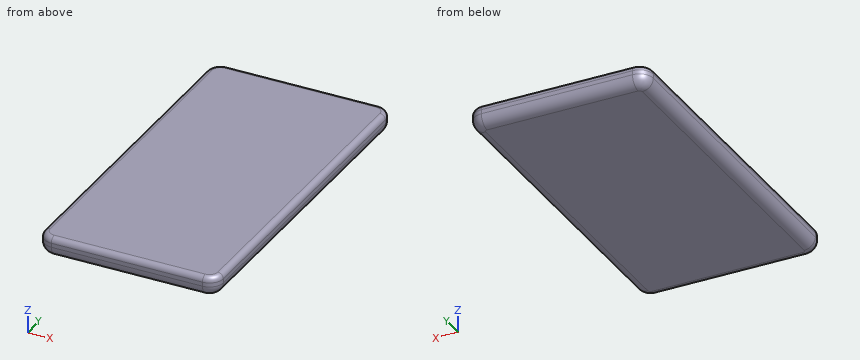
from build123d import *

# Parameters (mm, degrees)
F1_DEPTH = 9.525
F2_R     = 2.54
F3_R     = 5.08


with BuildPart() as f1:
    # F0 (on Top) → F1 (new body)
    with BuildSketch(Plane.XY):
        with BuildLine():
            Line((34.109328, 89.688999), (-35.740672, 89.688999))
            ThreePointArc((-35.740672, 89.688999), (-40.2308, 87.829127), (-42.090672, 83.338999))
            Line((-42.090672, 83.338999), (-42.090672, -62.711001))
            ThreePointArc((-42.090672, -62.711001), (-40.2308, -67.201129), (-35.740672, -69.061001))
            Line((-35.740672, -69.061001), (34.109328, -69.061001))
            ThreePointArc((34.109328, -69.061001), (38.599456, -67.201129), (40.459328, -62.711001))
            Line((40.459328, -62.711001), (40.459328, 83.338999))
            ThreePointArc((40.459328, 83.338999), (38.599456, 87.829127), (34.109328, 89.688999))
        make_face()
    extrude(amount=F1_DEPTH)

    # F2
    f2_edges = [f1.edges().sort_by_distance(p)[0] for p in [
        (-42.090672, 10.313999, 9.525),
        (-40.2308, -67.201129, 9.525),
        (-0.815672, -69.061001, 9.525),
        (38.599456, -67.201129, 9.525),
        (40.459328, 10.313999, 9.525),
        (38.599456, 87.829127, 9.525),
        (-0.815672, 89.688999, 9.525),
        (-40.2308, 87.829127, 9.525),
    ]]
    fillet(f2_edges, radius=F2_R)

    # F3
    f3_edges = [f1.edges().sort_by_distance(p)[0] for p in [
        (-42.090672, 10.313999, 0),
        (-40.2308, -67.201129, 0),
        (-0.815672, -69.061001, 0),
        (38.599456, -67.201129, 0),
        (40.459328, 10.313999, 0),
        (38.599456, 87.829127, 0),
        (-0.815672, 89.688999, 0),
        (-40.2308, 87.829127, 0),
    ]]
    fillet(f3_edges, radius=F3_R)


solid = f1.part
The listing builds one solid part. Answer for the finished solid, in the listing's coordinates (mm). Round coordinates to 2 decimals unless told otherwise and drop trailing zeros. Write each loop counter-clockwise with the first axis right and the second up, starting at its lowest first coordinate (ties: lowest second). Pieces come first, ordered by that corner, then holes. Notation, with made-up numbers: M -27.75,89.25 L -12.75,89.25 A16 cw -12.75,99.25 Z; hole C -12.75,66 d4. An arc over 180 degrees is marked long. Write each question's results on one line, items separated by ' | '. Start each with the question number.
(1) The part is cut by section A-A, the plane y = -0.5. Write down the section's boundary in (x, z) (3 decimals), and give its area (3 significant figures).
(2) This flat-tipped pin is pushed along its axis until it touches: P1, Ø2, axis at x = -20.5, z = 3, coming from the -Y side. Where does it stop, or does it pass through?
(3) Find the intervals of material crossed by line 1 (X direction, y = 65, z = 4.5); line 2 (Z direction, x = -37.5, y = 17) (3 decimals); line 3 (Y direction, x = 26, z = 1.25), in increasing order.
Worked answers:
1) outline: M -42.091,5.08 A5.08 ccw -37.011,0 L 35.379,0 A5.08 ccw 40.459,5.08 L 40.459,6.985 A2.54 ccw 37.919,9.525 L -39.551,9.525 A2.54 ccw -42.091,6.985 Z | area: 772 mm²
2) P1: stops at y = -68.94
3) line 1: x = -42.06 to 40.43 | line 2: z = 0.024 to 9.525 | line 3: y = -67.32 to 87.95
